```python
from build123d import *

# Parameters (mm, degrees)
F0_W     = 100
F0_H     = 250
F0_R     = 3.4
F0_R_2   = 4.25
F1_DEPTH = 6
F2_SIZE  = 0.5


with BuildPart() as f1:
    # F0 (on Right) → F1 (new body, symmetric)
    with BuildSketch(Plane.YZ):
        Rectangle(F0_W, F0_H)
        with Locations((-15, -102)):
            Circle(F0_R, mode=Mode.SUBTRACT)
        with Locations((-35, -51)):
            Circle(F0_R_2, mode=Mode.SUBTRACT)
        with Locations((15, -102)):
            Circle(F0_R, mode=Mode.SUBTRACT)
        with Locations((0, -51)):
            Circle(F0_R_2, mode=Mode.SUBTRACT)
        with Locations((35, -51)):
            Circle(F0_R_2, mode=Mode.SUBTRACT)
        with Locations((-15, 58)):
            Circle(F0_R, mode=Mode.SUBTRACT)
        with Locations((-35, 109)):
            Circle(F0_R_2, mode=Mode.SUBTRACT)
        with Locations((15, 58)):
            Circle(F0_R, mode=Mode.SUBTRACT)
        with Locations((0, 109)):
            Circle(F0_R_2, mode=Mode.SUBTRACT)
        with Locations((35, 109)):
            Circle(F0_R_2, mode=Mode.SUBTRACT)
    extrude(amount=F1_DEPTH, both=True)

    # F2
    f2_edges = [f1.edges().sort_by_distance(p)[0] for p in [
        (6, -39.25, 109),
        (0, -30.75, 109),
        (-6, -39.25, 109),
        (6, -4.25, 109),
        (0, 4.25, 109),
        (-6, -4.25, 109),
        (6, 30.75, 109),
        (0, 39.25, 109),
        (-6, 30.75, 109),
        (6, 30.75, -51),
        (0, 39.25, -51),
        (-6, 30.75, -51),
        (6, -4.25, -51),
        (0, 4.25, -51),
        (-6, -4.25, -51),
        (6, -39.25, -51),
        (0, -30.75, -51),
        (-6, -39.25, -51),
        (6, -18.4, 58),
        (0, -11.6, 58),
        (-6, -18.4, 58),
        (6, 11.6, 58),
        (0, 18.4, 58),
        (-6, 11.6, 58),
        (6, -18.4, -102),
        (0, -11.6, -102),
        (-6, -18.4, -102),
        (6, 11.6, -102),
        (0, 18.4, -102),
        (-6, 11.6, -102),
    ]]
    chamfer(f2_edges, length=F2_SIZE)


solid = f1.part
```
Can you work these out from the model? Positions are in its coordinate system, mm. Give positions to 0.01 mm unless a question says otherwise; leave off trailing zeros. Order: outer loops, then holes, each group sorted by start corner. A loop starts at its lowest first (then second) coordinate and runs counter-clockwise, first axis right, second up. Notation, with made-up numbers: (77, -15.5) - (81, -15.5) arc R14 cw to (81, 8.5) - close; hole circle Ø6 at (77, 88.25). An arc over 180 degrees is marked (long way). Use a Markdown table: item, result. Add a question column.
Q1. If we mould it in two halves opening along Y, with no side actions, what happens to faces 1 (the flat face through (0, 50, -2)), 2 (the flat face through (0, -1, 125)), 3 (the cylindrical face through (-0.1, -18.4, 58.1))? For each: released by +Y, released by -Y, zero draft, split by the parting line, or undercut.
Q2. If we section it at C-C on x = -1: Count the separate pieces of the cut face and the enclosed holes in it, plus the area to 3 significant figures.
Q3. Please list where these lines run through material, in increasing order: line 1 along Z through (x, y) = (-0.5, 0); line 2 along Z through (x, y) = (-0.25, -15); line 3 along Y through (x, z) = (5.5, -103).
Q4. If we section it at D-D on z = -51: Write out the boundary of the cut face in (x, y).
Q5. If we section it at B-B on z = -102: Write out the boundary of the cut face in (x, y), plus the area to 3 significant figures.
Q6. If we section it at A-A on y = -15: Write out the boundary of the cut face in (x, z).
Answers follow:
| question | item | result |
|---|---|---|
| 1 | face 1 | released by +Y |
| 1 | face 2 | zero draft |
| 1 | face 3 | undercut |
| 2 | separate pieces | 1 |
| 2 | enclosed holes | 10 |
| 2 | area | 24,500 mm^2 |
| 3 | line 1 | z = -125 to -55.25, -46.75 to 104.75, 113.25 to 125 |
| 3 | line 2 | z = -125 to -105.4, -98.6 to 54.6, 61.4 to 125 |
| 3 | line 3 | y = -50 to -18.25, -11.75 to 11.75, 18.25 to 50 |
| 4 | outline | (-6, -50) - (6, -50) - (6, -39.75) - (5.5, -39.25) - (-5.5, -39.25) - (-6, -39.75) - close; (-6, -30.25) - (-5.5, -30.75) - (5.5, -30.75) - (6, -30.25) - (6, -4.75) - (5.5, -4.25) - (-5.5, -4.25) - (-6, -4.75) - close; (-6, 4.75) - (-5.5, 4.25) - (5.5, 4.25) - (6, 4.75) - (6, 30.25) - (5.5, 30.75) - (-5.5, 30.75) - (-6, 30.25) - close; (-6, 39.75) - (-5.5, 39.25) - (5.5, 39.25) - (6, 39.75) - (6, 50) - (-6, 50) - close |
| 5 | outline | (-6, -50) - (6, -50) - (6, -18.9) - (5.5, -18.4) - (-5.5, -18.4) - (-6, -18.9) - close; (-6, -11.1) - (-5.5, -11.6) - (5.5, -11.6) - (6, -11.1) - (6, 11.1) - (5.5, 11.6) - (-5.5, 11.6) - (-6, 11.1) - close; (-6, 18.9) - (-5.5, 18.4) - (5.5, 18.4) - (6, 18.9) - (6, 50) - (-6, 50) - close |
| 5 | area | 1,040 mm^2 |
| 6 | outline | (-6, -125) - (6, -125) - (6, -105.9) - (5.5, -105.4) - (-5.5, -105.4) - (-6, -105.9) - close; (-6, -98.1) - (-5.5, -98.6) - (5.5, -98.6) - (6, -98.1) - (6, 54.1) - (5.5, 54.6) - (-5.5, 54.6) - (-6, 54.1) - close; (-6, 61.9) - (-5.5, 61.4) - (5.5, 61.4) - (6, 61.9) - (6, 125) - (-6, 125) - close |
